Source: CAD feature listing. Evaluate the final solid. Frame: model axes, mm. A direction names the side the tool comes from. Round coordinates to 2 decimals unless told otherwise and drop trailing zeros. Write each loop counter-clockwise with the first axis right and the second up, starting at its lowest first coordinate (ties: lowest second). Pieces come first, ordered by that corner, then holes. Notation, with made-up numbers: M -28,62.5 L -11,62.5 A22 cw -11,101.5 Z; hole C -4,58 d1. An arc over 180 degrees is marked long. Use a Markdown table: item, result.
```python
from build123d import *

# Parameters (mm, degrees)
SKETCH1_W                = 32.5
SKETCH1_H                = 26.5
BOSS_EXTRUDE1_DEPTH      = 1
SKETCH2_R                = 1
CUT_EXTRUDE1_DEPTH       = 2
BOSS_EXTRUDE3_DEPTH      = 0.1
BOSS_EXTRUDE3_DEPTH_BACK = 1.1
SKETCH3_R                = 2
SKETCH3_R_2              = 1


with BuildPart() as part:
    # Sketch1 → Boss-Extrude1 (new body)
    with BuildSketch(Plane.XY):
        Rectangle(SKETCH1_W, SKETCH1_H)
    extrude(amount=BOSS_EXTRUDE1_DEPTH)

    # Sketch2 → Cut-Extrude1 (cut)
    with BuildSketch(Plane.XY.offset(1)):
        with Locations((-13.75, 11.25)):
            Circle(SKETCH2_R)
        with Locations((-13.75, -2.75)):
            Circle(SKETCH2_R)
        with Locations((14.25, -2.75)):
            Circle(SKETCH2_R)
        with Locations((14.25, 11.25)):
            Circle(SKETCH2_R)
    extrude(amount=-CUT_EXTRUDE1_DEPTH, mode=Mode.SUBTRACT)

    # Sketch3 → Boss-Extrude3 (add, two sides: drawn at the far end of the back side and taken through both)
    # profile 1 of 4: a face of its own
    with BuildSketch(Plane.XY.offset(1).offset(-BOSS_EXTRUDE3_DEPTH_BACK)):
        with Locations((-13.75, 11.25)):
            Circle(SKETCH3_R)
        with Locations((-13.75, 11.25)):
            Circle(SKETCH3_R_2, mode=Mode.SUBTRACT)
    # profile 2 of 4: a face of its own
    with BuildSketch(Plane.XY.offset(1).offset(-BOSS_EXTRUDE3_DEPTH_BACK)):
        with Locations((14.25, 11.25)):
            Circle(SKETCH3_R)
        with Locations((14.25, 11.25)):
            Circle(SKETCH3_R_2, mode=Mode.SUBTRACT)
    # profile 3 of 4: a face of its own
    with BuildSketch(Plane.XY.offset(1).offset(-BOSS_EXTRUDE3_DEPTH_BACK)):
        with Locations((14.25, -2.75)):
            Circle(SKETCH3_R)
        with Locations((14.25, -2.75)):
            Circle(SKETCH3_R_2, mode=Mode.SUBTRACT)
    # profile 4 of 4: a face of its own
    with BuildSketch(Plane.XY.offset(1).offset(-BOSS_EXTRUDE3_DEPTH_BACK)):
        with Locations((-13.75, -2.75)):
            Circle(SKETCH3_R)
        with Locations((-13.75, -2.75)):
            Circle(SKETCH3_R_2, mode=Mode.SUBTRACT)
    extrude(amount=BOSS_EXTRUDE3_DEPTH + BOSS_EXTRUDE3_DEPTH_BACK)


solid = part.part
```
Q1. Reachability of faces 1 (the flat face through (16.25, -0.2, 0.5)), 2 (the flat face through (16, 13, 0)), 3 (the flat face through (16, 13, 1)) from +Z, -Z, +X, -X, +Y, -Y: full face, straight path, thin tool, end or side. Return the list, or none.
Results are:
| item | result |
|---|---|
| face 1 | +Z, -Z, +X, +Y, -Y |
| face 2 | -Z, +X, +Y |
| face 3 | +Z, +X, +Y |
Q2. Section B-B on x = 8.5. Return loops of the section in (y, z), plus the area to 3 significant figures.
Results are:
| item | result |
|---|---|
| outline | M -13.25,0 L 13.25,0 L 13.25,1 L -13.25,1 Z |
| area | 26.5 mm^2 |
Q3. First-contact query: pin 1 Ø1.8 at (x, y) = (14.25, -2.75) entering from +Z; pin 2 Ø13 at (x, y) = (1.5, -1) entering from +Z. Flat tips, straight axial feed; report the tip coordinate or a pass-through.
Results are:
| item | result |
|---|---|
| pin 1 | through |
| pin 2 | z = 1 |
Q4. Section A-A on y = -4.25. Return loops of the section in (x, z).
Results are:
| item | result |
|---|---|
| outline | M -16.25,0 L -15.07,0 L -15.07,-0.1 L -12.43,-0.1 L -12.43,0 L 12.93,0 L 12.93,-0.1 L 15.57,-0.1 L 15.57,0 L 16.25,0 L 16.25,1 L 15.57,1 L 15.57,1.1 L 12.93,1.1 L 12.93,1 L -12.43,1 L -12.43,1.1 L -15.07,1.1 L -15.07,1 L -16.25,1 Z |
Q5. Line query: L1, parallel to Y at x = 14.25, z = 0.9; L2, parallel to Z at x = 3, y = 10.5; L3, parallel to X at y = 10.5, z = 0.7. Output: solid intervals per line, ascending.
Results are:
| item | result |
|---|---|
| L1 | -13.25 to -3.75, -1.75 to 10.25, 12.25 to 13.25 |
| L2 | 0 to 1 |
| L3 | -16.25 to -14.41, -13.09 to 13.59, 14.91 to 16.25 |
Q6. Section C-C on y = 1.75. Return loops of the section in (x, z), plus the area to 3 significant figures.
Results are:
| item | result |
|---|---|
| outline | M -16.25,0 L 16.25,0 L 16.25,1 L -16.25,1 Z |
| area | 32.5 mm^2 |
